For this review, take the finished solid that the model builds, in its own axes (mm). A direction names the side the tool comes from. Give positions to 0.01 mm unless a question says otherwise; leave off trailing zeros. Loops run counter-clockwise (first coordinate to the right, second up) from the corner with the lowest first, then second, coordinate; pieces in that order, holes last.
```python
from build123d import *

# Parameters (mm, degrees)
BOSS_EXTRUDE1_DEPTH = 11.5
SKETCH1_13_R        = 1.5
SKETCH1_13_R_2      = 1.25
BOSS_EXTRUDE2_DEPTH = 8
BOSS_EXTRUDE3_DEPTH = 7


with BuildPart() as part:
    # Sketch1 → Boss-Extrude1 (new, symmetric)
    with BuildSketch(Plane(origin=(0, 0, 0), x_dir=(1, 0, 0), z_dir=(0, 1, 0))):
        with BuildLine():
            Line((6.824314586, 7.284360201), (6.824314586, 9.00020274))
            Line((6.824314586, 9.00020274), (-3.690467309, 9.00020274))
            Line((-3.690467309, 9.00020274), (-17.038497557, 11.5))
            Line((-17.038497557, 11.5), (-24.867971487, 11.5))
            Line((-24.867971487, 11.5), (-24.867971487, -11.5))
            Line((-24.867971487, -11.5), (-17.038497557, -11.5))
            Line((-17.038497557, -11.5), (-3.690467309, -9.00020274))
            Line((-3.690467309, -9.00020274), (6.824314586, -9.00020274))
            Line((6.824314586, -9.00020274), (6.824314586, -7.284360201))
            ThreePointArc((6.824314586, -7.284360201), (4.861171432, -6.879883717), (3.082035449, -5.956732906))
            Line((3.082035449, -5.956732906), (-3.422402494, -3.8))
            Line((-3.422402494, -3.8), (-19.513448301, -3.98254267))
            Line((-19.513448301, -3.98254267), (-19.513448301, 3.8))
            Line((-19.513448301, 3.8), (-3.422402494, 3.8))
            Line((-3.422402494, 3.8), (3.082035449, 5.956732906))
            ThreePointArc((3.082035449, 5.956732906), (4.861171432, 6.879883717), (6.824314586, 7.284360201))
        make_face()
    extrude(amount=BOSS_EXTRUDE1_DEPTH, both=True)

    # Sketch1<13> → Boss-Extrude2 (add, symmetric)
    with BuildSketch(Plane(origin=(0, 0, 0), x_dir=(1, 0, 0), z_dir=(0, 1, 0))):
        with BuildLine():
            Line((6.824314586, 3.971385595), (6.824314586, 7.284360201))
            ThreePointArc((6.824314586, 7.284360201), (4.861171432, 6.879883717), (3.082035449, 5.956732906))
            Line((3.082035449, 5.956732906), (-3.422402494, 3.8))
            Line((-3.422402494, 3.8), (-19.513448301, 3.8))
            Line((-19.513448301, 3.8), (-19.513448301, -3.98254267))
            Line((-19.513448301, -3.98254267), (-3.422402494, -3.8))
            Line((-3.422402494, -3.8), (3.082035449, -5.956732906))
            ThreePointArc((3.082035449, -5.956732906), (4.861171432, -6.879883717), (6.824314586, -7.284360201))
            Line((6.824314586, -7.284360201), (6.824314586, -3.971385595))
            ThreePointArc((6.824314586, -3.971385595), (3.301909035, 0), (6.824314586, 3.971385595))
        make_face()
        with Locations((-17.038497557, 0)):
            Circle(SKETCH1_13_R, mode=Mode.SUBTRACT)
        with Locations((-13.038497557, 0)):
            Circle(SKETCH1_13_R, mode=Mode.SUBTRACT)
        with Locations((-2.172402494, 0)):
            Circle(SKETCH1_13_R_2, mode=Mode.SUBTRACT)
    extrude(amount=BOSS_EXTRUDE2_DEPTH, both=True)

    # Sketch1<14> → Boss-Extrude3 (add, symmetric)
    with BuildSketch(Plane(origin=(0, 0, 0), x_dir=(1, 0, 0), z_dir=(0, 1, 0))):
        with BuildLine():
            Line((6.824314586, -3.971385595), (6.824314586, 3.971385595))
            ThreePointArc((6.824314586, 3.971385595), (3.301909035, 0), (6.824314586, -3.971385595))
        make_face()
    extrude(amount=BOSS_EXTRUDE3_DEPTH, both=True)


solid = part.part
```
Q1. Consider section C-C on y = 8.5. Give the boundary of the cut face in (x, z).
Answers:
outline: (-24.87, -11.5) - (-17.04, -11.5) - (-3.69, -9) - (6.82, -9) - (6.82, -7.28) arc R7.3 cw to (3.08, -5.96) - (-3.42, -3.8) - (-19.51, -3.8) - (-19.51, 3.98) - (-3.42, 3.8) - (3.08, 5.96) arc R7.3 cw to (6.82, 7.28) - (6.82, 9) - (-3.69, 9) - (-17.04, 11.5) - (-24.87, 11.5) - close
Q2. For pin 1 Ø3 at (x, y) = (2.5, 2.5) entering from +Z; pin 2 Ø1 at (y, z) = (10, 1) entering from +X; pin 3 Ø8.5 at (x, y) = (0, -3) entering from -Z (3 decimals); pin 4 Ø4.5 at (x, z) = (-10.5, -3) entering from +Y, all flat-tipped, find the tip position at first contact; note any pin that passes through.
Answers:
pin 1: stops at z = 9
pin 2: stops at x = -19.51
pin 3: stops at z = -9.105
pin 4: stops at y = 11.5
Q3. Consider section A-A on z = 0. Give the boundary of the cut face in (x, y), plus the area to 3 significant figures.
Answers:
outline: (-24.87, -11.5) - (-19.51, -11.5) - (-19.51, -8) - (-18.54, -8) - (-18.54, 8) - (-19.51, 8) - (-19.51, 11.5) - (-24.87, 11.5) - close; (-15.54, -8) - (-14.54, -8) - (-14.54, 8) - (-15.54, 8) - close; (-11.54, -8) - (-3.42, -8) - (-3.42, 8) - (-11.54, 8) - close; (-0.92, -8) - (3.3, -8) - (3.3, -7) - (6.82, -7) - (6.82, 7) - (3.3, 7) - (3.3, 8) - (-0.92, 8) - close
area: 402 mm2
Q4. Machinability: for faces 5 (the flat face through (-13, 11.5, 5)), 6 (the cylindrical face through (3.303, 7.507, 0.081)), 7 (the cylindrical face through (3.303, -7.493, 0.081)), which of the approach directions +Z, -Z, +X, -X, +Y, -Y give a long, thin tool a straight path to every point of the face, cutting with its end or side? Answer none if there is none.
Answers:
face 5: +Z, -Z, +X, -X, +Y
face 6: +X, +Y
face 7: +X, -Y
Q5. Mouldability with a two-part tool opening along Z and no side actions: class faces 1 (the flat face through (5, 7, 0)), 2 (the flat face through (2, 0, -9)), 3 (the flat face through (-24.868, 0, 0)), 4 (the flat face through (-7, -8, 0)) as +Z half, -Z half, draft (parallel to the pull), parting line (faces both ways), or undercut.
Answers:
face 1: undercut
face 2: -Z half
face 3: draft
face 4: undercut
Q6. For probe 1 along X at (y, z) = (0.25, 0); probe 2 along X at (y, z) = (1.5, -0.25); probe 3 along Z at (x, y) = (-0.5, 4), list the stretches that pass through material, from the lowest coordinate up.
Answers:
probe 1: x = -24.87 to -18.54, -15.54 to -14.54, -11.54 to -3.42, -0.92 to 6.82
probe 2: x = -24.87 to -18.52, -15.56 to -14.52, -11.56 to -3.4, -0.95 to 6.82
probe 3: z = -9 to 9
Q7. Consider section B-B on y = -3.75. Give the boundary of the cut face in (x, z).
Answers:
outline: (-24.87, -11.5) - (-17.04, -11.5) - (-3.69, -9) - (6.82, -9) - (6.82, 9) - (-3.69, 9) - (-17.04, 11.5) - (-24.87, 11.5) - close; hole circle Ø3 at (-17.04, 0); hole circle Ø3 at (-13.04, 0); hole circle Ø2.5 at (-2.17, 0)
Q8. Consider section D-D on x = -11. Give the boundary of the cut face in (y, z), plus the area to 3 significant figures.
Answers:
outline: (-11.5, -10.37) - (11.5, -10.37) - (11.5, -3.8) - (8, -3.8) - (8, 3.89) - (11.5, 3.89) - (11.5, 10.37) - (-11.5, 10.37) - (-11.5, 3.89) - (-8, 3.89) - (-8, -3.8) - (-11.5, -3.8) - close
area: 423 mm2
